from build123d import *

# Parameters (mm, degrees)
STOCK_PART1_1_START         = 40
STOCK_PART1_1_OUTLINE_W     = 90
STOCK_PART1_1_OUTLINE_H     = 55
STOCK_PART1_1_DEPTH         = 40
STOCK_PART1_1_START_2       = 75
STOCK_PART1_1_2_OUTLINE_W   = 90
STOCK_PART1_1_2_OUTLINE_H   = 55
STOCK_PART1_1_2_OUTLINE_R   = 6.10322586
STOCK_PART1_1_2_OUTLINE_R_2 = 17.5
STOCK_PART1_1_2_DEPTH       = 5
SKETCH1_W                   = 5
SKETCH1_H                   = 8.27683309
SKETCH1_W_2                 = 4.100738493
SKETCH1_H_2                 = 4.176305195
SKETCH1_W_3                 = 4.702811088
SKETCH1_H_3                 = 4.424974218
SKETCH1_W_4                 = 6.384187924
SKETCH1_H_4                 = 4.971555085
BOSS_EXTRUDE2_DEPTH         = 40
SKETCH2_W                   = 90
SKETCH2_H                   = 55
SKETCH2_W_2                 = 87.6
SKETCH2_H_2                 = 52.6
EXTRUDE_THIN1_DEPTH         = 35
SKETCH3_W                   = 89.6
SKETCH3_H                   = 54.6
SKETCH3_W_2                 = 87.6
SKETCH3_H_2                 = 52.6
EXTRUDE_THIN2_DEPTH         = 35
SKETCH4_R                   = 23.5
SKETCH4_R_2                 = 12.5
EXTRUDE_THIN3_DEPTH         = 5
SKETCH5_W                   = 54.6
SKETCH5_H                   = 27.201852287
CUT_EXTRUDE1_DEPTH          = 115


# Read off the part's stored shape, not the designer's step: Stock-Part1-1
with BuildPart() as part:
    # Stock-Part1-1 outline → Stock-Part1-1 (new body)
    with BuildSketch(Plane(origin=(0, 0, 0), x_dir=(1, 0, 0), z_dir=(0, 1, 0)).offset(STOCK_PART1_1_START)):
        with BuildLine():
            Line((55.93220339, -29.999229584), (55.93220339, 31.000770416))
            ThreePointArc((55.93220339, 31.000770416), (52.517989827, 29.586556854), (53.93220339, 33.000770416))
            Line((53.93220339, 33.000770416), (-42.06779661, 33.000770416))
            ThreePointArc((-42.06779661, 33.000770416), (-40.653583048, 29.586556854), (-44.06779661, 31.000770416))
            Line((-44.06779661, 31.000770416), (-44.06779661, -29.999229584))
            ThreePointArc((-44.06779661, -29.999229584), (-40.653583048, -28.585016022), (-42.06779661, -31.999229584))
            Line((-42.06779661, -31.999229584), (53.93220339, -31.999229584))
            ThreePointArc((53.93220339, -31.999229584), (52.517989827, -28.585016021), (55.93220339, -29.999229584))
        make_face()
        with Locations((5.93220339, 0.500770416)):
            Rectangle(STOCK_PART1_1_OUTLINE_W, STOCK_PART1_1_OUTLINE_H, mode=Mode.SUBTRACT)
    extrude(amount=STOCK_PART1_1_DEPTH)

    # Stock-Part1-1 2 outline → Stock-Part1-1 2 (add)
    with BuildSketch(Plane(origin=(0, 0, 0), x_dir=(1, 0, 0), z_dir=(0, 1, 0)).offset(STOCK_PART1_1_START_2)):
        with Locations((5.93220339, 0.500770416)):
            Rectangle(STOCK_PART1_1_2_OUTLINE_W, STOCK_PART1_1_2_OUTLINE_H)
        with Locations((36.155377847, 0)):
            Circle(STOCK_PART1_1_2_OUTLINE_R, mode=Mode.SUBTRACT)
        with Locations((-11.56779661, 0.500770416)):
            Circle(STOCK_PART1_1_2_OUTLINE_R_2, mode=Mode.SUBTRACT)
    extrude(amount=STOCK_PART1_1_2_DEPTH)

    # Sketch1 → Boss-Extrude2 (add)
    with BuildSketch(Plane.XZ.offset(-40)):
        with Locations((-41.56779661, -28.862353871)):
            Rectangle(SKETCH1_W, SKETCH1_H)
        with Locations((53.881834144, -30.912617819)):
            Rectangle(SKETCH1_W_2, SKETCH1_H_2)
        with Locations((53.580797846, 29.786742475)):
            Rectangle(SKETCH1_W_3, SKETCH1_H_3)
        with Locations((-40.875702648, 29.513452042)):
            Rectangle(SKETCH1_W_4, SKETCH1_H_4)
    extrude(amount=-BOSS_EXTRUDE2_DEPTH)

    # Sketch2 → Extrude-Thin1 (add)
    with BuildSketch(Plane.XZ.offset(-75)):
        with Locations((5.93220339, -0.500770416)):
            Rectangle(SKETCH2_W, SKETCH2_H)
        with Locations((5.93220339, -0.500770416)):
            Rectangle(SKETCH2_W_2, SKETCH2_H_2, mode=Mode.SUBTRACT)
    extrude(amount=EXTRUDE_THIN1_DEPTH)

    # Sketch3 → Extrude-Thin2 (add)
    with BuildSketch(Plane.XZ.offset(-40)):
        with Locations((5.93220339, -0.500770416)):
            Rectangle(SKETCH3_W, SKETCH3_H)
        with Locations((5.93220339, -0.500770416)):
            Rectangle(SKETCH3_W_2, SKETCH3_H_2, mode=Mode.SUBTRACT)
    extrude(amount=EXTRUDE_THIN2_DEPTH)

    # Sketch4 → Extrude-Thin3 (add)
    with BuildSketch(Plane(origin=(0, 80, 0), x_dir=(1, 0, 0), z_dir=(0, 1, 0))):
        with Locations((-11.56779661, 0.500770416)):
            Circle(SKETCH4_R)
        with Locations((-11.56779661, 0.500770416)):
            Circle(SKETCH4_R_2, mode=Mode.SUBTRACT)
    extrude(amount=-EXTRUDE_THIN3_DEPTH)

    # Sketch5 → Cut-Extrude1 (cut)
    with BuildSketch(Plane.ZY.offset(38.86779661)):
        with Locations((-0.500770416, 18.600926144)):
            Rectangle(SKETCH5_W, SKETCH5_H)
    extrude(amount=-CUT_EXTRUDE1_DEPTH, mode=Mode.SUBTRACT)


solid = part.part
Geometry check sheet. Reference: the model listing, model coordinates, mm. A direction names the side the tool comes from. Round coordinates to 2 decimals unless told otherwise and drop trailing zeros. Loops run counter-clockwise (first coordinate to the right, second up) from the corner with the lowest first, then second, coordinate; pieces in that order, holes last.
Item 1: Access from +Z, -Z, +X, -X, +Y, -Y to the whole of each face (thin tool, end or side, straight path). Record for faces 1 (the flat face through (-38.868, 36, -1)), 2 (the flat face through (-37.868, 54, -1)), 3 (the flat face through (5, 36, -27.801)).
Item 2: Thickness scan on line 1 (X direction, y = 78, z = 0); line 2 (Z direction, x = -12, y = 56.5); line 3 (X direction, y = 53, z = 18.5). Record the ranges inside material, lowest first.
Item 3: Cross-section at A-A on y = 65.5. Record the boundary of the cut face in (x, z).
Item 4: Gauge pin test, flat ends, axial feed: pin 1 (19.5 mm diameter, centred on x = 23, z = 5, fed in from -Y); pin 2 (2.5 mm diameter, centred on x = -8.5, y = 36, fed in from +Z); pin 3 (4 mm diameter, centred on y = 35, z = -13, fed in from +X). Record the tip position at first contact, or that the pin passes through.
Item 5: Mould release check, pull along X, two halves, no side actions. Record for faces 4 (the flat face through (5, 54, 25.799)), 5 (the flat face through (5, 80, 0)), 6 (the flat face through (50.732, 36, -1)): pulls with the +X half, pulls with the -X half, needs draft (parallel to the pull), parting line crosses it, or undercut.
Item 6: Cross-section at C-C on z = 21.5. Record the boundary of the cut face in (x, y), then the cut area to 3 significant figures.
Item 7: Cross-section at B-B on z = 10.5. Record the boundary of the cut face in (x, y), then the cut area to 3 significant figures.
Answer sheet:
1. face 1: +Z, -Z, -X, -Y
1. face 2: -Y
1. face 3: -Z, +X, -X, -Y
2. line 1: x = -44.07 to -24.06, 0.92 to 30.05, 42.26 to 55.93
2. line 2: z = -33 to -26.8, 25.8 to 32
2. line 3: x = -44.07 to -37.87, 49.73 to 55.93
3. outline: (-44.07, -33) - (55.93, -33) - (55.93, 32) - (-44.07, 32) - close; hole (-37.87, -26.8) - (49.73, -26.8) - (49.73, 25.8) - (-37.87, 25.8) - close
4. pin 1: stops at y = 75
4. pin 2: stops at z = 26.8
4. pin 3: stops at x = 50.73
5. face 4: undercut
5. face 5: needs draft
5. face 6: pulls with the +X half
6. outline: (-44.07, 40) - (-38.87, 40) - (-38.87, 32.2) - (-37.87, 32.2) - (-37.87, 75) - (49.73, 75) - (49.73, 32.2) - (50.73, 32.2) - (50.73, 40) - (55.93, 40) - (55.93, 80) - (-44.07, 80) - close
6. area: 950 mm2
7. outline: (-44.07, 40) - (-38.87, 40) - (-38.87, 32.2) - (-37.87, 32.2) - (-37.87, 75) - (-17.5, 75) - (-17.5, 80) - (-44.07, 80) - close; (-5.63, 75) - (49.73, 75) - (49.73, 32.2) - (50.73, 32.2) - (50.73, 40) - (55.93, 40) - (55.93, 80) - (-5.63, 80) - close
7. area: 890 mm2
